Verification items for the finished model (mm, model axes). Face numbers are marked on the shaded views. Give positions to 0.01 mm unless a question says otherwise; leave off trailing zeros. Loops run counter-clockwise (first coordinate to the right, second up) from the corner with the lowest first, then second, coordinate; pieces in that order, holes last. Notation, with made-up numbers: M 75,63.5 L 100,63.5 A21 ccw 100,86.5 Z; hole C -9,-6.75 d11. An arc over 180 degrees is marked long. Use CSV: the item, a comma, the result in double quotes.
from build123d import *

# Parameters (mm, degrees)
SKETCH1_W           = 14.732
SKETCH1_H           = 14.732
BOSS_EXTRUDE1_DEPTH = 25.4
SKETCH2_R           = 2.75
CUT_EXTRUDE1_DEPTH  = 31.272921564
SKETCH3_W           = 10
SKETCH3_H           = 6.858
SKETCH3_R           = 1.5875
CUT_EXTRUDE2_DEPTH  = 1.778
FILLET1_R           = 0.79375


with BuildPart() as part:
    # Sketch1 → Boss-Extrude1 (new body)
    with BuildSketch(Plane(origin=(0, 0, 0), x_dir=(0, 0, -1), z_dir=(1, 0, 0))):
        Rectangle(SKETCH1_W, SKETCH1_H)
    extrude(amount=BOSS_EXTRUDE1_DEPTH)

    # Sketch2 → Cut-Extrude1 (cut, through all)
    with BuildSketch(Plane(origin=(0, 7.366, 0), x_dir=(1, 0, 0), z_dir=(0, 1, 0))):
        with Locations(Location((12.7, 0, 0), (0, 0, 270))):
            Circle(SKETCH2_R)
    extrude(amount=-CUT_EXTRUDE1_DEPTH, mode=Mode.SUBTRACT)

    # Sketch3 → Cut-Extrude2 (cut)
    with BuildSketch(Plane(origin=(0, 0, -7.366), x_dir=(-1, 0, 0), z_dir=(0, 0, -1))):
        with Locations((-5, -0.063)):
            Rectangle(SKETCH3_W, SKETCH3_H)
        with Locations(Location((-4.92, -0.063, 0), (0, 0, 90))):
            Circle(SKETCH3_R, mode=Mode.SUBTRACT)
    extrude(amount=-CUT_EXTRUDE2_DEPTH, mode=Mode.SUBTRACT)

    # Fillet1
    fillet1_edges = [part.edges().sort_by_distance(p)[0] for p in [
        (10, -3.492, -6.477),
        (10, 3.366, -6.477),
    ]]
    fillet(fillet1_edges, radius=FILLET1_R)


solid = part.part
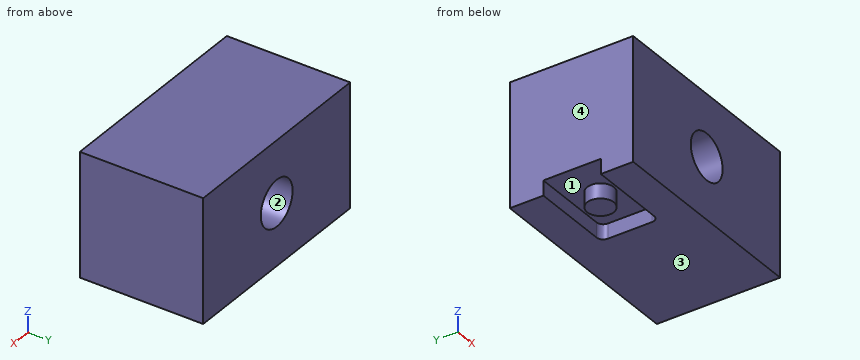
(1) Scan lines: L1, parallel to X at y = -2.75, z = 0; L2, parallel to X at y = 1, z = -1.25; L3, parallel to Z at x = 2.5, y = 0.25. Record each from-to range of solid material in increasing order. Write a range as from..to.
Calculated:
L1,"x = 0..9.95, 15.45..25.4"
L2,"x = 0..10.25, 15.15..25.4"
L3,"z = -5.59..7.37"
(2) Section check D-D on x = 4.92. Record the cut outline in (y, z), plus the area to 3 significant figures.
Calculated:
outline,"M -7.37,-7.37 L -3.49,-7.37 L -3.49,-5.59 L -1.65,-5.59 L -1.65,-7.37 L 1.52,-7.37 L 1.52,-5.59 L 3.37,-5.59 L 3.37,-7.37 L 7.37,-7.37 L 7.37,7.37 L -7.37,7.37 Z"
area,"210 mm²"
(3) Mould release check, pull along X, two halves, no side actions. Record for the marked faces 1, 2, 3 and 4: released by +X, released by -X, zero draft, split by the parting line, or undercut.
Calculated:
face 1,"undercut"
face 2,"undercut"
face 3,"zero draft"
face 4,"released by -X"
(4) Section check B-B on x = 12.7. Record the cut outline in (y, z).
Calculated:
outline,"M -7.37,-7.37 L 7.37,-7.37 L 7.37,-2.75 L -7.37,-2.75 Z; M -7.37,2.75 L 7.37,2.75 L 7.37,7.37 L -7.37,7.37 Z"
(5) Section check A-A on z = 0. Record the cut outline in (x, y), plus the area to 3 significant figures.
Calculated:
outline,"M 0,-7.37 L 9.95,-7.37 L 9.95,7.37 L 0,7.37 Z; M 15.45,-7.37 L 25.4,-7.37 L 25.4,7.37 L 15.45,7.37 Z"
area,"293 mm²"
(6) Section check C-C on y = -4. Record the cut outline in (x, z).
Calculated:
outline,"M 0,-7.37 L 25.4,-7.37 L 25.4,7.37 L 0,7.37 Z; hole C 12.7,0 d5.5"
